```python
from build123d import *

# Parameters (mm, degrees)
F0_W     = 79
F0_H     = 79
F1_DEPTH = 10
F2_W     = 49
F2_H     = 49
F3_DEPTH = 95


with BuildPart() as f1:
    # F0 (on Top) → F1 (new body)
    with BuildSketch(Plane.XY):
        Rectangle(F0_W, F0_H)
    extrude(amount=F1_DEPTH)

    # F2 (on face) → F3 (join)
    with BuildSketch(Plane.XY.offset(10)):
        Rectangle(F2_W, F2_H)
    extrude(amount=-F3_DEPTH)


solid = f1.part
```
Geometry: final body of the model. Coordinates: model frame, mm. A direction names the side the tool comes from. Coordinates: 2 decimals unless noted, no trailing zeros. Order: outer loops, then holes, each group sorted by start corner. A loop starts at its lowest first (then second) coordinate and runs counter-clockwise, first axis right, second up. Notation, with made-up numbers: (-5.75, -16.5) -> (47.25, -16.5) arc R16 cw to (47.25, 1.5) -> close; hole circle Ø3 at (-10.5, 32). An arc over 180 degrees is marked (long way). Use CSV: the item, a comma, the result in double quotes.
1) Access query for faces 4 (the flat face through (0, 24.5, -42)), 5 (the flat face through (-1, 39.5, 5)), 6 (the flat face through (-24.5, 0, -42)), 7 (the flat face through (24.5, 0, -42)), 8 (the flat face through (39.5, -1, 5)). Directions: +Z, -Z, +X, -X, +Y, -Y. A direction counts if a zero-diameter tool reaches every point of the face in a straight line with its end or side. Return the directions, or none.
Findings:
face 4,"-Z, +X, -X, +Y"
face 5,"+Z, -Z, +X, -X, +Y"
face 6,"-Z, -X, +Y, -Y"
face 7,"-Z, +X, +Y, -Y"
face 8,"+Z, -Z, +X, +Y, -Y"
2) Section C-C on z = -53.5. Output: boundary loops of the cut face in (x, y), then the cut area to 3 significant figures.
Findings:
outline,"(-24.5, -24.5) -> (24.5, -24.5) -> (24.5, 24.5) -> (-24.5, 24.5) -> close"
area,"2,400 mm^2"
3) Mould query, pull axis Z, two halves, no side actions, for faces 1 (the flat face through (-1, 1, 10)), 2 (the flat face through (0, -24.5, -42)), 3 (the flat face through (0, 0, -85)). Classes: +Z half, -Z half, draft (parallel to the pull), parting line (faces both ways), or undercut.
Findings:
face 1,"+Z half"
face 2,"draft"
face 3,"-Z half"
4) Section A-A on y = 2. Output: boundary loops of the cut face in (x, z), then the cut area to 4 significant figures.
Findings:
outline,"(-39.5, 0) -> (-24.5, 0) -> (-24.5, -85) -> (24.5, -85) -> (24.5, 0) -> (39.5, 0) -> (39.5, 10) -> (-39.5, 10) -> close"
area,"4,955 mm^2"
5) Line query: line 1 (Z direction, x = 25, y = 18.5); line 2 (Y direction, x = -10.5, z = -0.5). Output: solid intervals per line, ascending.
Findings:
line 1,"z = 0 to 10"
line 2,"y = -24.5 to 24.5"
6) Section D-D on y = 33. Output: boundary loops of the cut face in (x, z), then the cut area to 3 significant figures.
Findings:
outline,"(-39.5, 0) -> (39.5, 0) -> (39.5, 10) -> (-39.5, 10) -> close"
area,"790 mm^2"
7) Pin query (flat end, axial travel): pin 1 Ø4 at (y, z) = (-2.5, -56) entering from +X; pin 2 Ø1.5 at (x, z) = (7.5, -10.5) entering from -Y; pin 3 Ø5 at (x, y) = (-30.5, 12.5) entering from -Z. Return the tip coordinate at first contact, or that it passes through.
Findings:
pin 1,"stops at x = 24.5"
pin 2,"stops at y = -24.5"
pin 3,"stops at z = 0"
